```python
from build123d import *

# Parameters (mm, degrees)
BOSS_EXTRUDE1_DEPTH = 97.0775
SKETCH2_R           = 6.35
CUT_EXTRUDE1_DEPTH  = 22.08
CUT_EXTRUDE2_START  = -35
SKETCH3_R           = 6.35
CUT_EXTRUDE2_DEPTH  = 35
SKETCH4_W           = 9.525
SKETCH4_H           = 9.525
CUT_EXTRUDE3_DEPTH  = 12


with BuildPart() as part:
    # Sketch1 → Boss-Extrude1 (new body)
    with BuildSketch(Plane(origin=(0, 0, 0), x_dir=(1, 0, 0), z_dir=(0, 1, 0))):
        Polygon((5.499261314, 9.525), (-5.499261314, 9.525), (-10.998522628, 0), (-5.499261314, -9.525), (5.499261314, -9.525), (10.998522628, 0), align=None)
    extrude(amount=BOSS_EXTRUDE1_DEPTH)

    # Sketch2 → Cut-Extrude1 (cut)
    with BuildSketch(Plane(origin=(0, 97.0775, 0), x_dir=(1, 0, 0), z_dir=(0, 1, 0))):
        Polygon((10.998522628, 0), (5.499261314, 9.525), (-5.499261314, 9.525), (-10.998522628, 0), (-5.499261314, -9.525), (5.499261314, -9.525), align=None)
        with Locations(Location((0, 0, 0), (0, 0, 270))):
            Circle(SKETCH2_R, mode=Mode.SUBTRACT)
    extrude(amount=-CUT_EXTRUDE1_DEPTH, mode=Mode.SUBTRACT)

    # Sketch3 → Cut-Extrude2 (cut)
    with BuildSketch(Plane.XZ.offset(CUT_EXTRUDE2_START)):
        Polygon((5.499261314, -9.525), (10.998522628, 0), (5.499261314, 9.525), (-5.499261314, 9.525), (-10.998522628, 0), (-5.499261314, -9.525), align=None)
        with Locations(Location((0, 0, 0), (0, 0, 90))):
            Circle(SKETCH3_R, mode=Mode.SUBTRACT)
    extrude(amount=CUT_EXTRUDE2_DEPTH, mode=Mode.SUBTRACT)

    # Sketch4 → Cut-Extrude3 (cut)
    with BuildSketch(Plane.XZ):
        Polygon((-5.499261314, -9.525), (5.499261314, -9.525), (10.998522628, 0), (5.499261314, 9.525), (-5.499261314, 9.525), (-10.998522628, 0), align=None)
        Rectangle(SKETCH4_W, SKETCH4_H, mode=Mode.SUBTRACT)
    extrude(amount=-CUT_EXTRUDE3_DEPTH, mode=Mode.SUBTRACT)


solid = part.part
```
Verification items for the finished model (mm, model axes). A direction names the side the tool comes from. Coordinates: 2 decimals unless noted, no trailing zeros. Order: outer loops, then holes, each group sorted by start corner. A loop starts at its lowest first (then second) coordinate and runs counter-clockwise, first axis right, second up. Notation, with made-up numbers: (30, 65.25) -> (53, 65.25) arc R17 ccw to (53, 73.25) -> close; hole circle Ø2 at (22, 59.25). An arc over 180 degrees is marked (long way). Put each result on its own line as item: value. Start each with the question number.
1) Cross-section at C-C (z = -2). Enter the section's corners in (x, y), plus the area to 3 significant figures.
2) Cross-section at D-D (y = 71). Enter the section's corners in (x, z) (3 decimals), plus the area to 3 significant figures.
3) Tool access check on faces 1 (the flat face through (-0.2, 74.998, -6.5)), 2 (the flat face through (0, 6, -4.762)), 3 (the flat face through (0, 12, 5)), 4 (the flat face through (5, 12, 0)), 5 (the flat face through (-5, 12, 0)). Record the directions out of +Z, -Z, +X, -X, +Y, -Y that give a thin tool (end or side, any length) a straight path to the whole face; none if there is none.
4) Go/stop test with flat-tipped pins: pin 1 (2.5 mm diameter, centred on y = 6.5, z = 1, fed in from -X); pin 2 (1.7 mm diameter, centred on x = 5.5, z = -0.5, fed in from -Y); pin 3 (6.5 mm diameter, centred on y = 7.5, z = 1.5, fed in from +X); pin 4 (0.5 mm diameter, centred on x = -1, z = 5.5, fed in from -Y). Record where each tip stops, or that it passes through.
5) Cross-section at B-B (y = 7). Enter the section's corners in (x, z), plus the area to 3 significant figures.
6) Material ranges on L1, parallel to Y at x = -5, z = -6.5; L2, parallel to X at y = 20.5, z = -0.25; L3, parallel to Y at x = -0.75, z = 5.5, recorded low to high.
Geometry check:
1. outline: (-9.84, 35) -> (-6.03, 35) -> (-6.03, 12) -> (-4.76, 12) -> (-4.76, 0) -> (4.76, 0) -> (4.76, 12) -> (6.03, 12) -> (6.03, 35) -> (9.84, 35) -> (9.84, 75) -> (6.03, 75) -> (6.03, 97.08) -> (-6.03, 97.08) -> (-6.03, 75) -> (-9.84, 75) -> close
1. area: 1,450 mm^2
2. outline: (-10.999, 0) -> (-5.499, -9.525) -> (5.499, -9.525) -> (10.999, 0) -> (5.499, 9.525) -> (-5.499, 9.525) -> close
2. area: 314 mm^2
3. face 1: +Y
3. face 2: -Z, +X, -X, -Y
3. face 3: +Z, +X, -X, -Y
3. face 4: +Z, -Z, +X, -Y
3. face 5: +Z, -Z, -X, -Y
4. pin 1: stops at x = -4.76
4. pin 2: stops at y = 0
4. pin 3: stops at x = 4.76
4. pin 4: stops at y = 12
5. outline: (-4.76, -4.2) arc R6.35 ccw to (-4.2, -4.76) -> (4.2, -4.76) arc R6.35 ccw to (4.76, -4.2) -> (4.76, 4.2) arc R6.35 ccw to (4.2, 4.76) -> (-4.2, 4.76) arc R6.35 ccw to (-4.76, 4.2) -> close
5. area: 90.1 mm^2
6. L1: y = 35 to 75
6. L2: x = -6.35 to 6.35
6. L3: y = 12 to 97.08
